from build123d import *

# Parameters (mm, degrees)
EXTRUDE_1_DEPTH     = 15.1
EXTRUDE_1_2_DEPTH   = 15.1
SKETCH_1_W          = 55.05
SKETCH_1_H          = 4
EXTRUDE_1_3_DEPTH   = 15.1
SKETCH_2_W          = 4
SKETCH_2_H          = 16
SKETCH_2_W_2        = 19.05
EXTRUDE_2_DEPTH     = 4
EXTRUDE_3_DEPTH     = 20
SKETCH_4_R          = 1.8
CUT_EXTRUDE_1_DEPTH = 20
SKETCH_5_R          = 1.8
CUT_EXTRUDE_2_DEPTH = 27


with BuildPart() as part:
    # Sketch 1 → Extrude 1 (new body)
    with BuildSketch(Plane(origin=(0, 0, 0), x_dir=(1, 0, 0), z_dir=(0, 1, 0))):
        Polygon((-6.030769231, 9.384615385), (-22.030769231, 9.384615385), (-22.030769231, 5.384615385), (-6.030769231, 5.384615385), (-2.030769231, 5.384615385), (-2.030769231, 9.384615385), (-2.030769231, 25.384615385), (-6.030769231, 25.384615385), align=None)
    extrude(amount=EXTRUDE_1_DEPTH)



with BuildPart() as body_2:
    # Sketch 1 → Extrude 1 2 (new body)
    with BuildSketch(Plane(origin=(0, 0, 0), x_dir=(1, 0, 0), z_dir=(0, 1, 0))):
        Polygon((22.665384615, 5.384615385), (33.019230769, 5.384615385), (33.019230769, 9.384615385), (17.019230769, 9.384615385), (17.019230769, 25.384615385), (13.019230769, 25.384615385), (13.019230769, 8.769230769), (13.019230769, 5.384615385), align=None)
    extrude(amount=EXTRUDE_1_2_DEPTH)


with BuildPart() as body_3:
    # Sketch 1 → Extrude 1 3 (new body)
    with BuildSketch(Plane(origin=(0, 0, 0), x_dir=(1, 0, 0), z_dir=(0, 1, 0))):
        with Locations((5.494230769, -11.715384615)):
            Rectangle(SKETCH_1_W, SKETCH_1_H)
    extrude(amount=EXTRUDE_1_3_DEPTH)


with BuildPart() as part_1:
    add(part.part)

    add(body_2.part)  # Extrude 2 merges body 2

    add(body_3.part)  # Extrude 2 merges body 3
    # Sketch 2 → Extrude 2 (add)
    with BuildSketch(Plane(origin=(0, 15.1, 0), x_dir=(1, 0, 0), z_dir=(0, 1, 0))):
        with Locations((-4.030769231, 17.384615385)):
            Rectangle(SKETCH_2_W, SKETCH_2_H)
        with Locations((7.494230769, 17.384615385)):
            Rectangle(SKETCH_2_W_2, SKETCH_2_H)
        Polygon((-2.030769231, 5.384615385), (-22.030769231, 5.384615385), (-22.030769231, -13.715384615), (33.019230769, -13.715384615), (33.019230769, 9.384615385), (17.019230769, 9.384615385), (-2.030769231, 9.384615385), align=None)
        Polygon((-6.030769231, 9.384615385), (-22.030769231, 9.384615385), (-22.030769231, 5.384615385), (-2.030769231, 5.384615385), (-2.030769231, 9.384615385), align=None)
    extrude(amount=EXTRUDE_2_DEPTH)

    # Sketch 3 → Extrude 3 (add)
    with BuildSketch(Plane.XZ):
        Polygon((12.869230769, -9.384615385), (-5.980769231, -9.384615385), (-5.980769231, 13.715384615), (17.019230769, 13.715384615), (17.019230769, 9.715384615), (13.019230769, 9.715384615), (-2.130769231, 9.715384615), (-2.130769231, -5.384615385), (12.869230769, -5.384615385), align=None)
    extrude(amount=EXTRUDE_3_DEPTH)

    # Sketch 4 → Cut-Extrude 1 (cut)
    with BuildSketch(Plane(origin=(0, 19.1, 0), x_dir=(1, 0, 0), z_dir=(0, 1, 0))):
        with Locations((5.469230769, 17.884615385)):
            Circle(SKETCH_4_R)
        with Locations((5.469230769, -2.115384615)):
            Circle(SKETCH_4_R)
    extrude(amount=-CUT_EXTRUDE_1_DEPTH, mode=Mode.SUBTRACT)

    # Sketch 5 → Cut-Extrude 2 (cut)
    with BuildSketch(Plane.XY.offset(13.715384615)):
        with Locations((5.469230769, -12.5)):
            Circle(SKETCH_5_R)
    extrude(amount=-CUT_EXTRUDE_2_DEPTH, mode=Mode.SUBTRACT)


solid = part_1.part
CAD build for the part. Positions are in the model's coordinates, mm. A direction names the side the tool comes from. Give positions to 0.01 mm unless a question says otherwise; leave off trailing zeros. Write each loop counter-clockwise with the first axis right and the second up, starting at its lowest first coordinate (ties: lowest second). Pieces come first, ordered by that corner, then holes. Notation, with made-up numbers: M 6.5,72 L 34.5,72 A22 cw 34.5,95 Z; hole C -39.75,-18 d9. An arc over 180 degrees is marked long. Put each result on its own line as item: value. Start each with the question number.
(1) Band-saw the part on D-D, the plane z = -11. Write the cut outline in (x, y).
(2) Flat gauge pins, fed straight in: pin 1 Ø4.5 at (x, z) = (-13, 12.5) entering from -Y; pin 2 Ø1.2 at (y, z) = (-5, -7.5) entering from +X; pin 3 Ø1.5 at (y, z) = (-13, 9) entering from -X. Where does each tip first touch, or does it go through?
(3) Which spindle directions (+Z, -Z, +X, -X, +Y, -Y) get a long thin tool onto all of the face, cutting with end or side? Do faces 1 (the face through (17.019, 9, -17)), 2 (the face through (12.869, -10, -7)), 3 (the face through (7.186, 17.128, 1.575)), 4 (the face through (13.019, 7, -16)), 5 (the face through (-5.981, -10, 2)). Say none if no direction does.
(4) Mould opens along Y. For faces 6 (the face through (-2.131, -10, 2)), 7 (the face through (6, 0, -7)), 8 (the face through (-14, 0, 12)) say: +Y half, -Y half, draft (parallel to the pull), parting line (faces both ways), or undercut.
(5) Probe L1, parallel to Y at x = 12.5, z = -7; L2, parallel to Z at x = 19.5, y = 9.5; L3, parallel to X at y = 14, z = -16.5. List the from-to ranges inside material, lowest first.
(6) Band-saw the part on B-B, the plane y = -12.5. Write the cut outline in (x, z).
(7) Band-saw the part on C-C, the plane z = -3.5. Write the cut outline in (x, y), and give its area (3 significant figures).
(8) Band-saw the part on A-A, the plane x = 2. Write the cut outline in (y, z).
Response values:
1. outline: M -6.03,0 L -2.03,0 L -2.03,15.1 L 13.02,15.1 L 13.02,0 L 17.02,0 L 17.02,19.1 L -6.03,19.1 Z
2. pin 1: stops at y = 0
2. pin 2: stops at x = 12.87
2. pin 3: stops at x = -5.98
3. face 1: -Z, +X, +Y, -Y
3. face 2: -Z, +X, -Y
3. face 3: +Y, -Y
3. face 4: -Z, -Y
3. face 5: +Z, -Z, -X, -Y
4. face 6: draft
4. face 7: undercut
4. face 8: -Y half
5. L1: y = -20 to 0, 15.1 to 19.1
5. L2: z = -9.38 to -5.38, 9.72 to 13.72
5. L3: x = -6.03 to -2.03, 13.02 to 17.02
6. outline: M -5.98,-9.38 L 3.67,-9.38 L 3.67,-5.38 L -2.13,-5.38 L -2.13,9.72 L 3.67,9.72 L 3.67,13.72 L -5.98,13.72 Z; M 7.27,-9.38 L 12.87,-9.38 L 12.87,-5.38 L 7.27,-5.38 Z; M 7.27,9.72 L 17.02,9.72 L 17.02,13.72 L 7.27,13.72 Z
7. outline: M -22.03,15.1 L 33.02,15.1 L 33.02,19.1 L -22.03,19.1 Z; M -5.98,-20 L -2.13,-20 L -2.13,0 L -5.98,0 Z
7. area: 297 mm2
8. outline: M -20,-9.38 L 0,-9.38 L 0,-5.38 L -20,-5.38 Z; M -20,9.72 L 15.1,9.72 L 15.1,-25.38 L 19.1,-25.38 L 19.1,13.72 L -20,13.72 Z
